Design review of the part built by this model. Coordinates are the model's own, in mm. Face numbers are marked on the shaded views. A direction names the side the tool comes from. Coordinates: 2 decimals unless noted, no trailing zeros. Loops run counter-clockwise (first coordinate to the right, second up) from the corner with the lowest first, then second, coordinate; pieces in that order, holes last. Notation, with made-up numbers: (41, 7) -> (96, 7) arc R19 cw to (96, 25) -> close; hole circle Ø4 at (73, 59.5). An arc over 180 degrees is marked (long way). Answer as a JSON object with one key per item and string values.
```python
from build123d import *

# Parameters (mm, degrees)
SKETCH_1_W          = 40
SKETCH_1_H          = 20
EXTRUDE_1_DEPTH     = 6
SKETCH_2_R          = 2.5
CUT_EXTRUDE_1_DEPTH = 24.151673806
EXTRUDE_START       = -15
EXTRUDE_2_OUTLINE_R = 11
EXTRUDE_2_DEPTH     = 15
EXTRUDE_START_2     = -8
SKETCH_5_R          = 11
SKETCH_5_R_2        = 10
EXTRUDE_3_DEPTH     = 8
SKETCH_10_W         = 15
SKETCH_10_H         = 5
EXTRUDE_4_DEPTH     = 500
SKETCH_11_W         = 11.491200589
SKETCH_11_H         = 5.122583395
EXTRUDE_5_DEPTH     = 15
SKETCH_12_W         = 26.5
SKETCH_12_H         = 32
CUT_EXTRUDE_2_DEPTH = 481.59052217
SKETCH_14_W         = 424.807672393
SKETCH_14_H         = 21.861471412
CUT_EXTRUDE_3_DEPTH = 482.183177179
SKETCH_15_R         = 2.75
CUT_EXTRUDE_4_DEPTH = 10


# Read off the part's stored shape, not the designer's step: 凸台-拉伸2
with BuildPart() as part:
    # 草图1 → 凸台-拉伸1 (new body)
    with BuildSketch(Plane.XY):
        Rectangle(SKETCH_1_W, SKETCH_1_H)
    extrude(amount=EXTRUDE_1_DEPTH)

    # 草图2 → 切除-拉伸1 (cut, through all)
    with BuildSketch(Plane.XY.offset(6)):
        with Locations((10, 0)):
            Circle(SKETCH_2_R)
        with Locations((-1, 0)):
            Circle(SKETCH_2_R)
        with Locations((-12, 0)):
            Circle(SKETCH_2_R)
    extrude(amount=-CUT_EXTRUDE_1_DEPTH, mode=Mode.SUBTRACT)

    # 凸台-拉伸2 outline → 凸台-拉伸2 (add)
    with BuildSketch(Plane.XY.offset(6).offset(EXTRUDE_START)):
        with BuildLine():
            Line((20, 10), (20, 13.5))
            Line((20, 13.5), (-26.893967141, 13.5))
            Line((-26.893967141, 13.5), (-26.893967141, 13.384337644))
            ThreePointArc((-26.893967141, 13.384337644), (-45, 0), (-26.893967141, -13.384337644))
            Line((-26.893967141, -13.384337644), (-26.893967141, -13.5))
            Line((-26.893967141, -13.5), (20, -13.5))
            Line((20, -13.5), (20, -10))
            Line((20, -10), (-20, -10))
            Line((-20, -10), (-20, -8.660254038))
            ThreePointArc((-20, -8.660254038), (-17, 0), (-20, 8.660254038))
            Line((-20, 8.660254038), (-20, 10))
            Line((-20, 10), (20, 10))
        make_face()
        with Locations((-31, 0)):
            Circle(EXTRUDE_2_OUTLINE_R, mode=Mode.SUBTRACT)
    extrude(amount=EXTRUDE_2_DEPTH)

    # 草图5 → 凸台-拉伸3 (add)
    with BuildSketch(Plane.XY.offset(6).offset(EXTRUDE_START_2)):
        with Locations((-31, 0)):
            Circle(SKETCH_5_R)
        with Locations((-31, 0)):
            Circle(SKETCH_5_R_2, mode=Mode.SUBTRACT)
    extrude(amount=EXTRUDE_3_DEPTH)

    # 草图10 → 凸台-拉伸4 (add)
    with BuildSketch(Plane(origin=(20, 0, 0), x_dir=(0, 0, -1), z_dir=(1, 0, 0))):
        with Locations((1.5, -16)):
            Rectangle(SKETCH_10_W, SKETCH_10_H)
    extrude(amount=-EXTRUDE_4_DEPTH)

    # 草图11 → 凸台-拉伸5 (add, through all)
    with BuildSketch(Plane(origin=(0, 0, -9), x_dir=(-1, 0, 0), z_dir=(0, 0, -1))):
        with Locations((27.78271332, -13.925059853)):
            Rectangle(SKETCH_11_W, SKETCH_11_H)
    extrude(amount=-EXTRUDE_5_DEPTH)

    # 草图12 → 切除-拉伸2 (cut, through all)
    with BuildSketch(Plane.XY.offset(6)):
        with Locations((6.75, -2.5)):
            Rectangle(SKETCH_12_W, SKETCH_12_H)
    extrude(amount=-CUT_EXTRUDE_2_DEPTH, mode=Mode.SUBTRACT)

    # 草图14 → 切除-拉伸3 (cut, through all)
    with BuildSketch(Plane.XZ.offset(18.5)):
        with Locations((-281.623673677, 1.881654976)):
            Rectangle(SKETCH_14_W, SKETCH_14_H)
    extrude(amount=-CUT_EXTRUDE_3_DEPTH, mode=Mode.SUBTRACT)

    # 草图15 → 切除-拉伸4 (cut)
    with BuildSketch(Plane.XZ.offset(18.5)):
        with Locations(Location((-59.219837481, -1.5, 0), (0, 0, 270))):
            Circle(SKETCH_15_R)
    extrude(amount=-CUT_EXTRUDE_4_DEPTH, mode=Mode.SUBTRACT)


solid = part.part
```
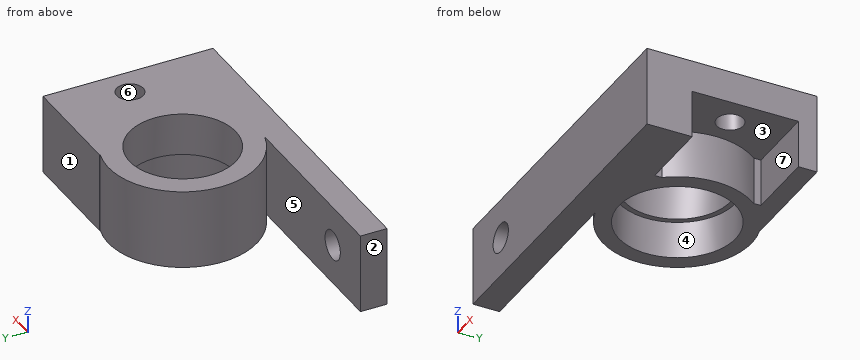
1) Wall thickness on probe 1 along X at (y, z) = (-16, -1.5); probe 2 along Y at (x, z) = (-31, -0.5); probe 3 along Y at (x, z) = (-14.5, -5.5): over which ranges is each line inside the solid? List them lowest first.
Completed:
{"probe 1": "-69.22 to -61.97, -56.47 to -6.5", "probe 2": "-18.5 to -10, 10 to 14", "probe 3": "-18.5 to -10, 10 to 13.5"}
2) The part is to be moulded in two halves that separate along Y. For the marked faces 1, 2 and 3, say which applies: pulls with the +Y half, pulls with the -Y half, needs draft (parallel to the pull), parting line crosses it, or undercut.
Completed:
{"face 1": "pulls with the +Y half", "face 2": "needs draft", "face 3": "undercut"}
3) Clearance check with flat-ended pins moving along their axes: pin 1 Ø3 at (y, z) = (1.5, 0.5) entering from -X; pin 2 Ø6 at (y, z) = (6.5, -5) entering from -X; pin 3 Ø4.5 at (x, z) = (-14, -1.5) entering from +Y; pin 4 Ø4.5 at (x, z) = (-59.22, -1.5) entering from +Y. State where each tip first meets the part, or that it passes through.
Completed:
{"pin 1": "x = -45", "pin 2": "x = -44.56", "pin 3": "y = 13.5", "pin 4": "through"}
4) Add section B-B, the plane y = 0. Give the boundary of the cut face in (x, z).
Completed:
{"outline": "(-45, -9) -> (-42, -9) -> (-42, -2) -> (-41, -2) -> (-41, 6) -> (-45, 6) -> close; (-21, -2) -> (-20, -2) -> (-20, -9) -> (-17, -9) -> (-17, 0) -> (-14.5, 0) -> (-14.5, 6) -> (-21, 6) -> close; (-9.5, 0) -> (-6.5, 0) -> (-6.5, 6) -> (-9.5, 6) -> close"}
5) Add section A-A, the plane x = -12. Give the boundary of the cut face in (y, z), and give its area (3 significant figures).
Completed:
{"outline": "(-18.5, -9) -> (-10, -9) -> (-10, 0) -> (-2.5, 0) -> (-2.5, 6) -> (-18.5, 6) -> close; (2.5, 0) -> (10, 0) -> (10, -9) -> (13.5, -9) -> (13.5, 6) -> (2.5, 6) -> close", "area": "270 mm²"}
6) Add section C-C, the plane z = 4.5. Give the boundary of the cut face in (x, y), and give its area (3 significant figures).
Completed:
{"outline": "(-69.22, -18.5) -> (-6.5, -18.5) -> (-6.5, 13.5) -> (-26.89, 13.5) -> (-26.89, 13.38) arc R14 ccw (long way) to (-34.71, -13.5) -> (-69.22, -13.5) -> close; hole circle Ø20 at (-31, 0); hole circle Ø5 at (-12, 0)", "area": "949 mm²"}
7) For the marked faces 4, 5, 6 and 7, list the 3-axis set-ups (+Z, -Z, +X, -X, +Y, -Y) from which the entire face can be reached by the end or side of a thin tool; tool diameter is ignored.
Completed:
{"face 4": "-Z", "face 5": "+Z, -Z, -X", "face 6": "+Z, -Z", "face 7": "-Z, +X"}
8) Add section D-D, the plane x = -40. Give the boundary of the cut face in (y, z), and give its area (3 significant figures).
Completed:
{"outline": "(-18.5, -9) -> (-13.5, -9) -> (-13.5, 6) -> (-18.5, 6) -> close; (-10.72, -9) -> (-6.32, -9) -> (-6.32, -2) -> (-4.36, -2) -> (-4.36, 6) -> (-10.72, 6) -> close; (4.36, -2) -> (6.32, -2) -> (6.32, -9) -> (10.72, -9) -> (10.72, 6) -> (4.36, 6) -> close", "area": "238 mm²"}
